Autodesk Inventor part; units mm, degrees
ref_plane "YZ Plane" through (0, 0, 0) normal (1, 0, 0) x (0, 1, 0)
ref_plane "XZ Plane" through (0, 0, 0) normal (0, 1, 0) x (-1, 0, 0)
ref_plane "XY Plane" through (0, 0, 0) normal (0, 0, 1) x (1, 0, 0)
sketch "スケッチ1" plane through (0, 0, 0) normal (0, 1, 0) x (-1, 0, 0)
  line L0 (97.5, 15) -> (-97.5, 15)
  line L1 (-97.5, 15) -> (-97.5, -15)
  line L2 (-97.5, -15) -> (97.5, -15)
  line L3 (97.5, -15) -> (97.5, 15)
  line L4 (97.5, 15) -> (-97.5, -15) construction
  line L5 (-97.5, 15) -> (97.5, -15) construction
  point P0 (0, 0)
  dimension "d0" = 195
  dimension "d1" = 30
extrude "プレート1" add sketch "スケッチ1" along normal blind 2
sketch "スケッチ2" plane through (0, 2, 0) normal (0, 1, 0) x (1, 0, 0)
  line L0 (-14, -5) -> (34.6, -5)
  line L1 (34.6, -5) -> (34.6, 5)
  line L2 (34.6, 5) -> (-14, 5)
  line L3 (-14, 5) -> (-14, -5)
  line L4 (-14, -5) -> (34.6, 5) construction
  line L5 (34.6, -5) -> (-14, 5) construction
  point P0 (0, 0)
  point P1 (10.3, 0)
  point P2 (10.3, 0)
  dimension "d3" = 48.6
  dimension "d4" = 14
  dimension "d5" = 10
hole "穴1" at (34.6, 2, -5) at (34.6, 2, 5) at (-14, 2, -5) at (-14, 2, 5) direction (0, -1, 0) diameter 4.3 end through all
sketch "スケッチ3" plane through (0, 2, 0) normal (0, 1, 0) x (1, 0, 0)
  circle A0 centre (0, 0) radius 6
  dimension "d13" = 12
extrude "押し出し1" cut sketch "スケッチ3" against normal through all
sketch "スケッチ4" plane through (0, 2, 0) normal (0, 1, 0) x (1, 0, 0)
  line L0 (97.5, 15) -> (97.5, -15)
  line L1 (-97.5, 15) -> (97.5, 15)
  line L2 (97.5, -15) -> (-97.5, -15)
  line L3 (-97.5, -15) -> (-97.5, 15)
  point P0 (0, 0)
  point P1 (-92.5, 10)
  point P2 (-92.5, -10)
  point P3 (92.5, 10)
  point P4 (92.5, -10)
  dimension "d16" = 5
  dimension "d17" = 5
  dimension "d18" = 5
  dimension "d19" = 5
hole "穴2" at (-92.5, 2, -10) at (-92.5, 2, 10) at (92.5, 2, -10) at (92.5, 2, 10) direction (0, -1, 0) diameter 3.2 end through all
equation "\"d11\" = Thickness"
equation "\"d25\" = Thickness"
equation "\"d2\" = Thickness"
equation "\"BendRadius\" = Thickness"
equation "\"BendReliefWidth\" = Thickness"
equation "\"BendReliefDepth\" = 0.5 * Thickness"
equation "\"CornerReliefSize\" = 4 * Thickness"
equation "\"MinimumRemnant\" = 2 * Thickness"
equation "\"TransitionRadius\" = BendRadius"
equation "\"JacobiRadiusSize\" = BendRadius"
equation "\"GapSize\" = Thickness"
properties part number "s_carbon_plate3"
Input: part model. Units: mm. Frame: model coordinates. Give positions to 0.01 mm unless a question says otherwise; leave off trailing zeros. Write each loop counter-clockwise with the first axis right and the second up, starting at its lowest first coordinate (ties: lowest second). Pieces come first, ordered by that corner, then holes.
Q1. Material intervals for probe 1 along Z at (x, y) = (34.6, 0.95); probe 2 along X at (y, z) = (0.8, -10); probe 3 along X at (y, z) = (1.25, 5.5), sorted ascending.
Q2. Section C-C, the plane x = -14. Output: boundary loops of the cut face in (y, z).
Q3. Pull-direction query (Z, two-part tool) for faces 1 (the face through (92.43, 0.99, -11.6)), 2 (the face through (1, 0, 7)); classes: pulls with the +Z half, pulls with the -Z half, needs draft (parallel to the pull), parting line crosses it, or undercut.
Q4. Section D-D, the plane z = 10. Output: boundary loops of the cut face in (x, y).
Q5. Section B-B, the plane y = 1.5. State how many separate pieces and enclosed holes the cut face has, plus the area to 3 significant figures.
Q6. Section A-A, the plane z = 0. Output: boundary loops of the cut face in (x, y).
Filled in:
1. probe 1: z = -15 to -7.15, -2.85 to 2.85, 7.15 to 15
1. probe 2: x = -97.5 to -94.1, -90.9 to 90.9, 94.1 to 97.5
1. probe 3: x = -97.5 to -16.09, -11.91 to -2.4, 2.4 to 32.51, 36.69 to 97.5
2. outline: (0, -15) - (2, -15) - (2, -7.15) - (0, -7.15) - close; (0, -2.85) - (2, -2.85) - (2, 2.85) - (0, 2.85) - close; (0, 7.15) - (2, 7.15) - (2, 15) - (0, 15) - close
3. face 1: undercut
3. face 2: needs draft
4. outline: (-97.5, 0) - (-94.1, 0) - (-94.1, 2) - (-97.5, 2) - close; (-90.9, 0) - (90.9, 0) - (90.9, 2) - (-90.9, 2) - close; (94.1, 0) - (97.5, 0) - (97.5, 2) - (94.1, 2) - close
5. separate pieces: 1
5. enclosed holes: 9
5. area: 5,650 mm2
6. outline: (-97.5, 0) - (-6, 0) - (-6, 2) - (-97.5, 2) - close; (6, 0) - (97.5, 0) - (97.5, 2) - (6, 2) - close
